from build123d import *

# Parameters (mm, degrees)
SALIENTE_EXTRUIR1_DEPTH = 50
SALIENTE_EXTRUIR2_DEPTH = 50
SALIENTE_EXTRUIR3_DEPTH = 50
CORTAR_EXTRUIR1_DEPTH   = 30
CROQUIS8_W              = 25.4
CROQUIS8_H              = 25.4
CORTAR_EXTRUIR5_DEPTH   = 50
CROQUIS9_W              = 25.4
CROQUIS9_H              = 25.4
CORTAR_EXTRUIR6_DEPTH   = 50
CORTAR_EXTRUIR7_DEPTH   = 50
CORTAR_EXTRUIR8_DEPTH   = 50
CORTAR_EXTRUIR9_DEPTH   = 50


with BuildPart() as part:
    # Croquis1 → Revolución1 (revolve)
    with BuildSketch(Plane.XY):
        with BuildLine():
            Line((0, 25.4), (0, -25.4))
            ThreePointArc((0, -25.4), (25.4, 0), (0, 25.4))
        make_face()
    revolve(axis=Axis((0, 32.899125747, 0), (0, -1, 0)))

    # Croquis2 → Saliente-Extruir1 (add)
    with BuildSketch(Plane(origin=(0, 0, 0), x_dir=(1, 0, 0), z_dir=(0, 1, 0))):
        with BuildLine():
            Line((0, 25.4), (0, 0))
            Line((0, 0), (25.4, 0))
            ThreePointArc((25.4, 0), (17.960512242, 17.960512242), (0, 25.4))
        make_face()
    extrude(amount=SALIENTE_EXTRUIR1_DEPTH)

    # Croquis3 → Saliente-Extruir2 (add)
    with BuildSketch(Plane.XY):
        with BuildLine():
            Line((0, 0), (25.4, 0))
            ThreePointArc((25.4, 0), (17.960512242, -17.960512242), (0, -25.4))
            Line((0, -25.4), (0, 0))
        make_face()
    extrude(amount=SALIENTE_EXTRUIR2_DEPTH)

    # Croquis4 → Saliente-Extruir3 (add)
    with BuildSketch(Plane(origin=(0, 0, 0), x_dir=(0, 0, -1), z_dir=(1, 0, 0))):
        with BuildLine():
            Line((25.4, 0), (0, 0))
            Line((0, 0), (0, -25.4))
            ThreePointArc((0, -25.4), (17.960512242, -17.960512242), (25.4, 0))
        make_face()
    extrude(amount=-SALIENTE_EXTRUIR3_DEPTH)

    # Croquis5 → Cortar-Extruir1 (cut, symmetric)
    with BuildSketch(Plane.XY):
        with BuildLine():
            Line((0, 25.4), (0, 0))
            Line((0, 0), (-25.4, 0))
            ThreePointArc((-25.4, 0), (-17.960512242, 17.960512242), (0, 25.4))
        make_face()
    extrude(amount=CORTAR_EXTRUIR1_DEPTH, both=True, mode=Mode.SUBTRACT)

    # Croquis8 → Cortar-Extruir5 (cut)
    with BuildSketch(Plane(origin=(0, 0, 0), x_dir=(0, 0, -1), z_dir=(1, 0, 0))):
        with Locations((-12.7, 12.7)):
            Rectangle(CROQUIS8_W, CROQUIS8_H)
    extrude(amount=CORTAR_EXTRUIR5_DEPTH, mode=Mode.SUBTRACT)

    # Croquis9 → Cortar-Extruir6 (cut)
    with BuildSketch(Plane(origin=(0, 0, 0), x_dir=(1, 0, 0), z_dir=(0, 1, 0))):
        with Locations((-12.7, -12.7)):
            Rectangle(CROQUIS9_W, CROQUIS9_H)
    extrude(amount=-CORTAR_EXTRUIR6_DEPTH, mode=Mode.SUBTRACT)

    # Croquis11 → Cortar-Extruir7 (cut)
    with BuildSketch(Plane.ZY.offset(50)):
        with BuildLine():
            Line((0, -25.4), (0, 0))
            Line((0, 0), (-25.4, 0))
            ThreePointArc((-25.4, 0), (-17.960512242, -17.960512242), (0, -25.4))
        make_face()
        with BuildLine():
            Line((-1, -24.379499585), (-1, -1))
            Line((-1, -1), (-24.379499585, -1))
            ThreePointArc((-24.379499585, -1), (-17.253405461, -17.253405461), (-1, -24.379499585))
        make_face(mode=Mode.SUBTRACT)
    extrude(amount=-CORTAR_EXTRUIR7_DEPTH, mode=Mode.SUBTRACT)

    # Croquis12 → Cortar-Extruir8 (cut)
    with BuildSketch(Plane(origin=(0, 50, 0), x_dir=(1, 0, 0), z_dir=(0, 1, 0))):
        with BuildLine():
            Line((0, 25.4), (0, 0))
            Line((0, 0), (25.4, 0))
            ThreePointArc((25.4, 0), (17.960512242, 17.960512242), (0, 25.4))
        make_face()
        with BuildLine():
            Line((1, 24.379499585), (1, 1))
            Line((1, 1), (24.379499585, 1))
            ThreePointArc((24.379499585, 1), (17.253405461, 17.253405461), (1, 24.379499585))
        make_face(mode=Mode.SUBTRACT)
    extrude(amount=-CORTAR_EXTRUIR8_DEPTH, mode=Mode.SUBTRACT)

    # Croquis13 → Cortar-Extruir9 (cut)
    with BuildSketch(Plane.XY.offset(50)):
        with BuildLine():
            Line((0, 0), (0, -25.4))
            ThreePointArc((0, -25.4), (17.960512242, -17.960512242), (25.4, 0))
            Line((25.4, 0), (0, 0))
        make_face()
        with BuildLine():
            Line((1, -1), (1, -24.379499585))
            ThreePointArc((1, -24.379499585), (17.253405461, -17.253405461), (24.379499585, -1))
            Line((24.379499585, -1), (1, -1))
        make_face(mode=Mode.SUBTRACT)
    extrude(amount=-CORTAR_EXTRUIR9_DEPTH, mode=Mode.SUBTRACT)


solid = part.part
Work out the finished part from the listing and answer in its coordinate system (mm). A direction names the side the tool comes from. Give positions to 0.01 mm unless a question says otherwise; leave off trailing zeros. Order: outer loops, then holes, each group sorted by start corner. A loop starts at its lowest first (then second) coordinate and runs counter-clockwise, first axis right, second up. Notation, with made-up numbers: (-28, 14) - (22, 14) arc R27 cw to (22, 47) - close; hole circle Ø11 at (-38, 70.5). An arc over 180 degrees is marked (long way). Answer as CSV lines item,"result". Start each with the question number.
Q1. Find the intervals of material crossed by L1, parallel to Z at x = -13.5, y = -13.5; L2, parallel to Y at x = -10, z = -19.5; L3, parallel to Z at x = 9.5, y = -21.5, in increasing order. Write a range as [from, to].
Q2. The part is cut by section B-B (y = -13.5). Write down the section's boundary in (x, z), then the cut area to 3 significant figures.
Q3. Given pin 1 Ø18.5 at (y, z) = (22.5, -13) entering from -X; pin 2 Ø11.5 at (x, y) = (14, 29) entering from +Z; pin 3 Ø5 at (y, z) = (-4, 42) entering from +X, each flat-ended and moving along its own axis, determine where each tip first touches the part or whether it passes through.
Q4. The part is cut by section A-A (x = 15.5). Write down the section's boundary in (y, z).
Q5. For faces 1 (the face through (17.073, -17.432, 25.35)), 2 (the face through (-25, -13, -1)), 3 (the face through (13, -1, 25)), 4 (the face through (-25, -1, -13)), 5 (the face through (17.432, 25.35, -17.073)), determine the directions among +Z, -Z, +X, -X, +Y, -Y from which every point of the face is accessible in a straight line to the end or side of a thin tool.
Q6. The part is cut by section C-C (z = 21). Write down the section's boundary in (x, y), then the cut area to 3 significant figures.
Check result:
1,L1,"z = [-20.33, -1]"
1,L2,"y = [-14.67, -1]"
1,L3,"z = [-9.63, 50]"
2,outline,"(-50, -20.33) - (0, -20.33) - (0, -21.52) arc R21.52 ccw to (21.52, 0) - (20.33, 0) - (20.33, 50) - (1, 50) - (1, 0) - (0, 0) - (0, -1) - (-50, -1) - close"
2,area,"2,300 mm²"
3,pin 1,"stops at x = 1"
3,pin 2,"stops at z = -1"
3,pin 3,"stops at x = 24.35"
4,outline,"(-20.12, 0) arc R20.12 ccw to (0, -20.12) - (0, -18.84) - (50, -18.84) - (50, -1) - (0, -1) - (0, 0) - (-1, 0) - (-1, 50) - (-18.84, 50) - (-18.84, 0) - close"
5,face 1,"+Z, +X, -Y"
5,face 2,"+Z, -X, +Y, -Y"
5,face 3,"+Z, +X, -X, +Y"
5,face 4,"+Z, -Z, -X, +Y"
5,face 5,"-Z, +X, +Y"
6,outline,"(1, -24.38) arc R24.4 ccw to (24.38, -1) - (1, -1) - close"
6,area,"420 mm²"
